```python
from build123d import *

# Parameters (mm, degrees)
SKETCH1_W           = 73
SKETCH1_H           = 62
BOSS_EXTRUDE1_DEPTH = 0.75
CUT_EXTRUDE1_DEPTH  = 2
SKETCH3_R           = 1.5
CUT_EXTRUDE2_DEPTH  = 2
SKETCH4_W           = 6
SKETCH4_H           = 42
SKETCH4_H_2         = 52
SKETCH4_W_2         = 2
SKETCH4_H_3         = 15
SKETCH4_H_4         = 20
BOSS_EXTRUDE2_DEPTH = 9
CHAMFER1_SIZE       = 1.5
SKETCH5_W           = 2
SKETCH5_H           = 15
BOSS_EXTRUDE3_DEPTH = 2
SKETCH6_W           = 2
SKETCH6_H           = 20
BOSS_EXTRUDE4_DEPTH = 2


with BuildPart() as part:
    # Sketch1 → Boss-Extrude1 (new, symmetric)
    with BuildSketch(Plane(origin=(0, 0, 0), x_dir=(1, 0, 0), z_dir=(0, 1, 0))):
        Rectangle(SKETCH1_W, SKETCH1_H)
    extrude(amount=BOSS_EXTRUDE1_DEPTH, both=True)

    # Sketch2 → Cut-Extrude1 (cut)
    with BuildSketch(Plane(origin=(0, 0.75, 0), x_dir=(1, 0, 0), z_dir=(0, 1, 0))):
        Polygon((-36.5, -31), (-36.5, -28), (-23.5, -28), (-20.5, -31), align=None)
        Polygon((36.5, -31), (12.5, -31), (14.5, -28), (36.5, -28), align=None)
    extrude(amount=-CUT_EXTRUDE1_DEPTH, mode=Mode.SUBTRACT)

    # Sketch3 → Cut-Extrude2 (cut)
    with BuildSketch(Plane(origin=(0, 0.75, 0), x_dir=(1, 0, 0), z_dir=(0, 1, 0))):
        with Locations(Location((-17.5, -28.5, 0), (0, 0, 270))):
            Circle(SKETCH3_R)
        with Locations(Location((9.5, -28.5, 0), (0, 0, 90))):
            Circle(SKETCH3_R)
        with Locations(Location((24.5, 22, 0), (0, 0, 270))):
            Circle(SKETCH3_R)
    extrude(amount=-CUT_EXTRUDE2_DEPTH, mode=Mode.SUBTRACT)

    # Sketch4 → Boss-Extrude2 (add)
    with BuildSketch(Plane(origin=(0, 0.75, 0), x_dir=(1, 0, 0), z_dir=(0, 1, 0))):
        with Locations((-31.5, -4)):
            Rectangle(SKETCH4_W, SKETCH4_H)
        with Locations((31.5, 1)):
            Rectangle(SKETCH4_W, SKETCH4_H_2)
        with Locations((-25.5, -1.5)):
            Rectangle(SKETCH4_W_2, SKETCH4_H_3)
        with Locations((-25.5, -18.5)):
            Rectangle(SKETCH4_W_2, SKETCH4_H_3)
        with Locations((22.5, 6)):
            Rectangle(SKETCH4_W_2, SKETCH4_H_4)
        with Locations((22.5, -16)):
            Rectangle(SKETCH4_W_2, SKETCH4_H_4)
    extrude(amount=BOSS_EXTRUDE2_DEPTH)

    # Chamfer1
    chamfer1_edges = [part.edges().sort_by_distance(p)[0] for p in [
        (-34.5, 9.75, 4),
        (-28.5, 9.75, 4),
        (34.5, 9.75, -1),
        (28.5, 9.75, -1),
    ]]
    chamfer(chamfer1_edges, length=CHAMFER1_SIZE)

    # Sketch5 → Boss-Extrude3 (add)
    with BuildSketch(Plane.XZ.offset(0.75)):
        with Locations((-23.5, 18.5)):
            Rectangle(SKETCH5_W, SKETCH5_H)
        with Locations((-23.5, 1.5)):
            Rectangle(SKETCH5_W, SKETCH5_H)
    extrude(amount=BOSS_EXTRUDE3_DEPTH)

    # Sketch6 → Boss-Extrude4 (add)
    with BuildSketch(Plane.XZ.offset(0.75)):
        with Locations((24.5, 16)):
            Rectangle(SKETCH6_W, SKETCH6_H)
        with Locations((24.5, -6)):
            Rectangle(SKETCH6_W, SKETCH6_H)
    extrude(amount=BOSS_EXTRUDE4_DEPTH)


solid = part.part
```
Verification items for the finished model (mm, model axes). A direction names the side the tool comes from. Coordinates: 2 decimals unless noted, no trailing zeros. Loops run counter-clockwise (first coordinate to the right, second up) from the corner with the lowest first, then second, coordinate; pieces in that order, holes last. Notation, with made-up numbers: (-36.5, 66.5) - (-21.5, 66.5) arc R17 ccw to (-21.5, 83.5) - close; hole circle Ø9 at (45.5, 75.25). An arc over 180 degrees is marked (long way). Put each result on its own line as item: value.
Item 1: Set-up check for faces 4 (the face through (24, -2, 4)), 5 (the face through (-24.5, -2, 1)), 6 (the face through (-24, -2, 11)): record each of +Z, -Z, +X, -X, +Y, -Y from which the full face is reachable in a straight line by a thin tool's end or side.
Conclusion:
face 4: +X, -Y
face 5: +Z, -Z, -X, -Y
face 6: -X, -Y
Item 2: Section check C-C (x = 9.5). Enter the section's corners in (y, z).
Conclusion:
outline: (-0.75, -31) - (0.75, -31) - (0.75, 27) - (-0.75, 27) - close; (-0.75, 30) - (0.75, 30) - (0.75, 31) - (-0.75, 31) - close
Item 3: Section check A-A (z = -22). Enter the section's corners in (x, y), then the cut area to 3 significant figures.
Conclusion:
outline: (-36.5, -0.75) - (23, -0.75) - (23, 0.75) - (-36.5, 0.75) - close; (26, -0.75) - (36.5, -0.75) - (36.5, 0.75) - (34.5, 0.75) - (34.5, 8.25) - (33, 9.75) - (30, 9.75) - (28.5, 8.25) - (28.5, 0.75) - (26, 0.75) - close
area: 157 mm2
Item 4: Section check B-B (y = 2.25). Enter the section's corners in (x, z).
Conclusion:
outline: (-34.5, -17) - (-28.5, -17) - (-28.5, 25) - (-34.5, 25) - close; (-26.5, -6) - (-24.5, -6) - (-24.5, 9) - (-26.5, 9) - close; (-26.5, 11) - (-24.5, 11) - (-24.5, 26) - (-26.5, 26) - close; (21.5, -16) - (23.5, -16) - (23.5, 4) - (21.5, 4) - close; (21.5, 6) - (23.5, 6) - (23.5, 26) - (21.5, 26) - close; (28.5, -27) - (34.5, -27) - (34.5, 25) - (28.5, 25) - close
Item 5: Scan lines: line 1 along X through (y, z) = (5.5, -2.5); line 2 along X through (y, z) = (5, -12.5); line 3 along X through (y, z) = (-1.25, 2.5). Record each from-to range of solid material in increasing order.
Conclusion:
line 1: x = -34.5 to -28.5, -26.5 to -24.5, 21.5 to 23.5, 28.5 to 34.5
line 2: x = -34.5 to -28.5, 21.5 to 23.5, 28.5 to 34.5
line 3: x = -24.5 to -22.5, 23.5 to 25.5
Item 6: Draft check along X on faces 1 (the face through (-1, 0.75, 0)), 2 (the face through (22, 9.75, -6)), 3 (the face through (-36.5, 0, -1)). Enter one of: pulls with the +X half, pulls with the -X half, needs draft (parallel to the pull), parting line crosses it, or undercut.
Conclusion:
face 1: undercut
face 2: needs draft
face 3: pulls with the -X half
Item 7: Gauge pin test, flat ends, axial feed: pin 1 Ø1 at (x, z) = (1.5, 20.5) entering from +Y; pin 2 Ø1.6 at (x, y) = (-29.5, 0.5) entering from +Z; pin 3 Ø2 at (x, y) = (-29, -1) entering from -Z; pin 4 Ø7 at (y, z) = (6.5, 17.5) entering from -X. Record the tip position at first contact, or that the pin passes through.
Conclusion:
pin 1: stops at y = 0.75
pin 2: stops at z = 28
pin 3: stops at z = -31
pin 4: stops at x = -34.5
